For this review, take the finished solid that the model builds, in its own axes (mm). Give positions to 0.01 mm unless a question says otherwise; leave off trailing zeros. Order: outer loops, then holes, each group sorted by start corner. A loop starts at its lowest first (then second) coordinate and runs counter-clockwise, first axis right, second up. Notation, with made-up numbers: (51, 55) -> (103, 55) arc R12 ccw to (103, 73) -> close; hole circle Ø9 at (-33.5, 13.5). An arc over 180 degrees is marked (long way). Return JSON: item names as keys, results as strings. Group by question number.
1) Add section C-C (x = -79.5). Give the boundary of the cut face in (y, z).
2) Add section D-D (z = -26). Give the boundary of the cut face in (x, y).
3) To check wall thickness, follow line 1 along X through (y, z) = (2.9, -31.5); line 2 along X through (y, z) = (2.2, -25.25); line 3 along X through (y, z) = (1.25, -27). State the ranges of each line that lie inside material, in increasing order.
4) Add section A-A (z = -29.5). Give the boundary of the cut face in (x, y), then the cut area to 3 significant figures.
5) Add section B-B (y = 1.2). State how many separate pieces and enclosed holes the cut face has, then the cut area to 3 significant figures.
6) Insertion check: P1, Ø2, axis at x = -69.5, y = 2, coming from the +Z side; P2, Ø2, axis at y = 3, z = -26.5, coming from the +X side; P3, Ø1.2, axis at y = 2, z = -25.5, coming from the -X side. Each pin has a flat end and moves straight along its axis. Give the tip position at first contact, or say it passes through.
Autodesk Inventor part; units mm, degrees
ref_plane "YZ Plane" through (0, 0, 0) normal (1, 0, 0) x (0, 1, 0)
ref_plane "XZ Plane" through (0, 0, 0) normal (0, 1, 0) x (-1, 0, 0)
ref_plane "XY Plane" through (0, 0, 0) normal (0, 0, 1) x (1, 0, 0)
sketch "Sketch1" plane through (0, 0, 0) normal (0, 1, 0) x (-1, 0, 0)
  line L0 (26.0651, -39.5603) -> (116.0651, -39.5603)
  line L1 (116.0651, -39.5603) -> (116.0651, -27.5603)
  line L2 (116.0651, -27.5603) -> (26.0651, -27.5603)
  line L3 (26.0651, -27.5603) -> (26.0651, -39.5603)
  line L4 (39.5651, -27.5603) -> (47.5651, -27.5603)
  line L5 (47.5651, -27.5603) -> (47.5651, -21.5603)
  line L6 (47.5651, -21.5603) -> (39.5651, -21.5603)
  line L7 (39.5651, -21.5603) -> (39.5651, -27.5603)
  line L8 (69.5651, -27.5603) -> (77.5651, -27.5603)
  line L9 (77.5651, -27.5603) -> (77.5651, -21.5603)
  line L10 (77.5651, -21.5603) -> (69.5651, -21.5603)
  line L11 (69.5651, -21.5603) -> (69.5651, -27.5603)
  line L12 (99.5651, -27.5603) -> (107.5651, -27.5603)
  line L13 (107.5651, -27.5603) -> (107.5651, -21.5603)
  line L14 (107.5651, -21.5603) -> (99.5651, -21.5603)
  line L15 (99.5651, -21.5603) -> (99.5651, -27.5603)
  point P0 (0, 0)
  dimension "d0" = 90
  dimension "d3" = 12
  dimension "d4" = 21.5
  dimension "d5" = 30
  dimension "d6" = 30
  dimension "d7" = 6
  dimension "d8" = 6
  dimension "d9" = 6
  dimension "d10" = 8
  dimension "d11" = 8
  dimension "d12" = 8
extrude "Extrusion1" add sketch "Sketch1" along normal blind 5
fillet "Fillet1" radius 2 1 edges at (-99.5651, 2.5, -21.5603)
fillet "Fillet2" radius 2 1 edges at (-107.5651, 2.5, -21.5603)
fillet "Fillet3" radius 2 1 edges at (-77.5651, 2.5, -21.5603)
fillet "Fillet4" radius 2 1 edges at (-69.5651, 2.5, -21.5603)
fillet "Fillet5" radius 2 1 edges at (-47.5651, 2.5, -21.5603)
fillet "Fillet6" radius 2 1 edges at (-39.5651, 2.5, -21.5603)
sketch "Sketch2" plane through (0, 0, 0) normal (0, -1, 0) x (1, 0, 0)
  line L0 (-39.5651, -23.5603) -> (-39.5651, -27.5603)
  circle A0 centre (-103.5651, -25.0603) radius 1.75
  circle A1 centre (-73.5651, -25.0603) radius 1.75
  circle A2 centre (-43.5651, -25.0603) radius 1.75
  line L1 (-69.5651, -27.5603) -> (-47.5651, -27.5603)
  line L2 (-69.5651, -23.5603) -> (-69.5651, -27.5603)
  line L3 (-99.5651, -27.5603) -> (-77.5651, -27.5603)
  line L4 (-99.5651, -23.5603) -> (-99.5651, -27.5603)
  line L5 (-39.5651, -27.5603) -> (-26.0651, -27.5603)
  point P0 (0, 0)
  dimension "d23" = 3.5
  dimension "d29" = 3.5
  dimension "d30" = 3.5
  dimension "d47" = 2.5
  dimension "d48" = 4
  dimension "d49" = 2.5
  dimension "d50" = 4
  dimension "d51" = 2.5
  dimension "d52" = 4
extrude "Extrusion2" cut sketch "Sketch2" against normal blind 10
sketch "Sketch4" plane through (0, 5, 0) normal (0, 1, 0) x (1, 0, 0)
  line L0 (-26.0651, 27.5603) -> (-26.0651, 39.5603)
  line L1 (-26.0651, 39.5603) -> (-116.0651, 39.5603)
  line L2 (-116.0651, 39.5603) -> (-116.0651, 27.5603)
  arc A0 (-108.5651, 34.5603) -> (-113.5651, 34.5603) centre (-111.0651, 34.5603) ccw
  arc A1 (-28.5651, 34.5603) -> (-33.5651, 34.5603) centre (-31.0651, 34.5603) ccw
  line L3 (-113.5651, 27.5603) -> (-108.5651, 27.5603)
  line L4 (-108.5651, 27.5603) -> (-108.5651, 34.5603)
  line L5 (-113.5651, 34.5603) -> (-113.5651, 27.5603)
  line L6 (-33.5651, 27.5603) -> (-28.5651, 27.5603)
  line L7 (-28.5651, 27.5603) -> (-28.5651, 34.5603)
  line L8 (-33.5651, 34.5603) -> (-33.5651, 27.5603)
  line L9 (-39.5651, 27.5603) -> (-26.0651, 27.5603)
  line L10 (-116.0651, 27.5603) -> (-107.5651, 27.5603)
  point P0 (0, 0)
  dimension "d53" = 5
  dimension "d54" = 5
  dimension "d55" = 5
  dimension "d56" = 5
  dimension "d57" = 5
  dimension "d58" = 5
extrude "Extrusion4" cut sketch "Sketch4" against normal blind 10
equation "\"d8\" = d7"
equation "\"d9\" = d7"
properties part number "RodHolderV4" material "Copper"
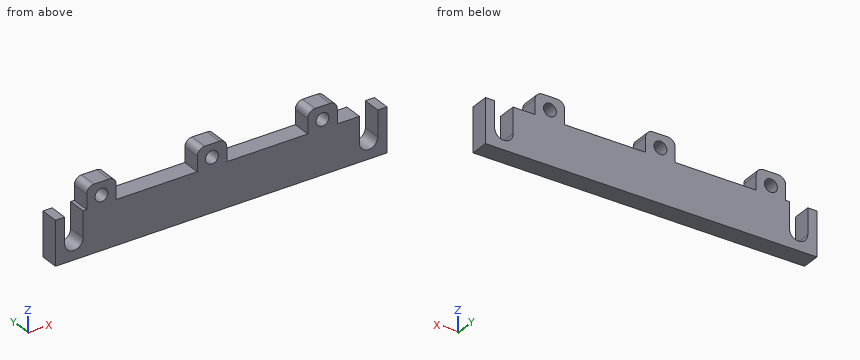
Evaluation:
{
 "1": {"outline": "(0, -39.56) -> (5, -39.56) -> (5, -27.56) -> (0, -27.56) -> close"},
 "2": {"outline": "(-107.57, 0) -> (-105.04, 0) -> (-105.04, 5) -> (-107.57, 5) -> close; (-102.09, 0) -> (-99.57, 0) -> (-99.57, 5) -> (-102.09, 5) -> close; (-77.57, 0) -> (-75.04, 0) -> (-75.04, 5) -> (-77.57, 5) -> close; (-72.09, 0) -> (-69.57, 0) -> (-69.57, 5) -> (-72.09, 5) -> close; (-47.57, 0) -> (-45.04, 0) -> (-45.04, 5) -> (-47.57, 5) -> close; (-42.09, 0) -> (-39.57, 0) -> (-39.57, 5) -> (-42.09, 5) -> close"},
 "3": {"line 1": "-116.07 to -113.57, -108.57 to -33.57, -28.57 to -26.07", "line 2": "-107.57 to -105.3, -101.83 to -99.57, -77.57 to -75.3, -71.83 to -69.57, -47.57 to -45.3, -41.83 to -39.57", "line 3": "-107.57 to -99.57, -77.57 to -69.57, -47.57 to -39.57"},
 "4": {"outline": "(-116.07, 0) -> (-113.57, 0) -> (-113.57, 5) -> (-116.07, 5) -> close; (-108.57, 0) -> (-33.57, 0) -> (-33.57, 5) -> (-108.57, 5) -> close; (-28.57, 0) -> (-26.07, 0) -> (-26.07, 5) -> (-28.57, 5) -> close", "area": "400 mm^2"},
 "5": {"separate pieces": "1", "enclosed holes": "3", "area": "1,100 mm^2"},
 "6": {"P1": "z = -21.87", "P2": "x = -39.57", "P3": "x = -107.57"}
}
